Can you work these out from the model? Positions are in its coordinate system, mm. A direction names the side the tool comes from. Round coordinates to 2 decimals unless told otherwise and drop trailing zeros. Order: outer loops, then holes, each group sorted by start corner. A loop starts at its lowest first (then second) coordinate and runs counter-clockwise, first axis right, second up.
Q1. Will these pins go through, and if not, where does the flat tip stop? P1, Ø2, axis at x = -15, z = 0, coming from the -Y side; P2, Ø4, axis at x = 22, z = 0, coming from the -Y side; P3, Ø3, axis at x = -20.5, z = 0.5, coming from the -Y side; P4, Ø5, axis at x = -12, z = 24, coming from the -Y side.
Q2. We'd pull the mould along Z, two halves only. Please class faces 1 (the face through (-9, 18.5, -13)), 2 (the face through (-12, -17, 0)): pulls with the +Z half, pulls with the -Z half, needs draft (parallel to the pull), parting line crosses it, or undercut.
Q3. For faces 3 (the face through (21.57, 17.49, -0.65)), 4 (the face through (-12.436, 15.451, 15.94)), 5 (the face through (-7, -15.5, 7)), which set-ups out of +Z, -Z, +X, -X, +Y, -Y let a thin tool reach every point of the face, with its end or its side?
Q4. If I drill on line 1 (Z direction, x = 0, y = -16); line 2 (Z direction, x = 10, y = 18.1); line 3 (Y direction, x = -12.5, z = 8), over which ranges is the centre line in solid material (lowest first)?
Q5. If we section it at C-C (y = -4): Please give me the cut outline in (x, z).
Q6. If we section it at B-B (x = 0): Please give me the cut outline in (y, z).
Q7. If we section it at D-D (z = -22): Count the separate pieces of the cut face and the enclosed holes in it, plus the area to 3 significant figures.
Q8. If we section it at A-A (y = 4.5): Please give me the cut outline in (x, z), plus the area to 3 significant figures.
from build123d import *

# Parameters (mm, degrees)
SKETCH_W              = 76
SKETCH_H              = 37
PAD_DEPTH             = 30
SKETCH020_R           = 14
POCKET_DEPTH          = 8
SKETCH026_R           = 1.7
PAD001_DEPTH          = 2
POCKET001_DEPTH       = 4
POLARPATTERN_COUNT    = 6
SKETCH025_R           = 1.7
POCKET005_DEPTH       = 211.317184
POLARPATTERN001_COUNT = 6
SKETCH022_R           = 1.7
SKETCH022_R_2         = 7
SKETCH022_W           = 3.5
SKETCH022_H           = 5
POCKET002_DEPTH       = 5
SKETCH027_W           = 5
SKETCH027_H           = 30
POCKET006_DEPTH       = 4.001
SKETCH028_R           = 1.6
POCKET007_DEPTH       = 5
POCKET008_DEPTH       = 2
FILLET_R              = 7
FILLET001_R           = 7
FILLET002_R           = 5
FILLET003_R           = 5
FILLET004_R           = 3
FILLET005_R           = 3
FILLET006_R           = 3
FILLET007_R           = 3
FILLET008_R           = 2
FILLET009_R           = 2
CHAMFER_SIZE          = 1.7
CHAMFER001_SIZE       = 1.7
CHAMFER002_SIZE       = 1.7
CHAMFER003_SIZE       = 1.7


with BuildPart() as part:
    # Sketch → Pad (new body, symmetric)
    with BuildSketch(Plane.XY):
        Rectangle(SKETCH_W, SKETCH_H)
        Polygon((-34, -11.5), (-30, -15.5), (30, -15.5), (34, -11.5), (34, 12.5), (12.5, 14.5), (-12.5, 14.5), (-34, 12.5), align=None, mode=Mode.SUBTRACT)
    extrude(amount=PAD_DEPTH, both=True)

    # Sketch020 → Pocket (cut)
    with BuildSketch(Plane(origin=(0, 18.5, 0), x_dir=(-1, 0, 0), z_dir=(0, 1, 0))):
        Circle(SKETCH020_R)
    extrude(amount=-POCKET_DEPTH, mode=Mode.SUBTRACT)

    # Sketch026 → Pad001 (new body)
    with BuildSketch(Plane.XZ.offset(-14.5)):
        with Locations((20, 0)):
            Circle(SKETCH026_R)
    extrude(amount=PAD001_DEPTH)

    # Sketch021 → Pocket001 (cut)
    with BuildSketch(Plane.XZ.offset(-12.5)):
        Polygon((18.383419, 2.8), (16.766838, 0), (18.383419, -2.8), (21.616581, -2.8), (23.233162, 0), (21.616581, 2.8), align=None)
    pocket001 = extrude(amount=-POCKET001_DEPTH, mode=Mode.SUBTRACT)

    # PolarPattern: Pocket001 ×6 about axis
    polarpattern_axis = Axis((0, 12.5, 0), (0, -1, 0))
    for i in range(1, POLARPATTERN_COUNT):
        add(pocket001.rotate(polarpattern_axis, i * 360 / POLARPATTERN_COUNT), mode=Mode.SUBTRACT)

    # Sketch025 → Pocket005 (cut, through all)
    with BuildSketch(Plane.XZ.offset(-14.5)):
        with Locations((20, 0)):
            Circle(SKETCH025_R)
    pocket005 = extrude(amount=-POCKET005_DEPTH, mode=Mode.SUBTRACT)

    # PolarPattern001: Pocket005 ×6 about axis
    polarpattern001_axis = Axis((0, 14.5, 0), (0, -1, 0))
    for i in range(1, POLARPATTERN001_COUNT):
        add(pocket005.rotate(polarpattern001_axis, i * 360 / POLARPATTERN001_COUNT), mode=Mode.SUBTRACT)

    # Sketch022 → Pocket002 (cut)
    with BuildSketch(Plane.XZ.offset(18.5)):
        with Locations((0, 22)):
            Circle(SKETCH022_R)
        with Locations((0, -22)):
            Circle(SKETCH022_R)
        with Locations((-22, 0)):
            Circle(SKETCH022_R)
        with Locations((22, 0)):
            Circle(SKETCH022_R)
        Circle(SKETCH022_R_2)
        with Locations((-15, 0)):
            Circle(SKETCH022_R)
        with BuildLine():
            ThreePointArc((-23.660997, 14.014536), (-21.731705, 6.47943), (-14.196598, 8.408722))
            ThreePointArc((-8.408722, 14.196598), (-11.667262, 11.667262), (-14.196598, 8.408722))
            ThreePointArc((-8.408722, 14.196598), (-6.47943, 21.731705), (-14.014536, 23.660997))
            ThreePointArc((-14.014536, 23.660997), (-19.445436, 19.445436), (-23.660997, 14.014536))
        make_face()
        with BuildLine():
            ThreePointArc((8.408722, -14.196598), (11.667262, -11.667262), (14.196598, -8.408722))
            ThreePointArc((23.660997, -14.014536), (21.731705, -6.47943), (14.196598, -8.408722))
            ThreePointArc((14.014536, -23.660997), (19.445436, -19.445436), (23.660997, -14.014536))
            ThreePointArc((8.408722, -14.196598), (6.47943, -21.731705), (14.014536, -23.660997))
        make_face()
        with BuildLine():
            ThreePointArc((23.660997, 14.014536), (19.445436, 19.445436), (14.014536, 23.660997))
            ThreePointArc((14.014536, 23.660997), (6.47943, 21.731705), (8.408722, 14.196598))
            ThreePointArc((14.196598, 8.408722), (11.667262, 11.667262), (8.408722, 14.196598))
            ThreePointArc((14.196598, 8.408722), (21.731705, 6.47943), (23.660997, 14.014536))
        make_face()
        with BuildLine():
            ThreePointArc((-14.014536, -23.660997), (-6.47943, -21.731705), (-8.408722, -14.196598))
            ThreePointArc((-14.196598, -8.408722), (-11.667262, -11.667262), (-8.408722, -14.196598))
            ThreePointArc((-14.196598, -8.408722), (-21.731705, -6.47943), (-23.660997, -14.014536))
            ThreePointArc((-23.660997, -14.014536), (-19.445436, -19.445436), (-14.014536, -23.660997))
        make_face()
        with Locations((-10.25, 0)):
            Rectangle(SKETCH022_W, SKETCH022_H)
    extrude(amount=-POCKET002_DEPTH, mode=Mode.SUBTRACT)

    # Sketch027 → Pocket006 (cut, through all)
    with BuildSketch(Plane.XZ.offset(-14.5)):
        with Locations((0, 15)):
            Rectangle(SKETCH027_W, SKETCH027_H)
    extrude(amount=-POCKET006_DEPTH, mode=Mode.SUBTRACT)

    # Sketch028 → Pocket007 (cut)
    with BuildSketch(Plane(origin=(-38, 0, 0), x_dir=(0, -1, 0), z_dir=(-1, 0, 0))):
        with Locations((4, 17.5)):
            Circle(SKETCH028_R)
        with Locations((4, -17.5)):
            Circle(SKETCH028_R)
        with BuildLine():
            ThreePointArc((11, 5), (4, 12), (-3, 5))
            Line((-3, 5), (-3, -5))
            ThreePointArc((-3, -5), (4, -12), (11, -5))
            Line((11, 5), (11, -5))
        make_face()
    extrude(amount=-POCKET007_DEPTH, mode=Mode.SUBTRACT)

    # Sketch029 → Pocket008 (cut)
    with BuildSketch(Plane.YZ.offset(-34)):
        Polygon((-2.383419, 14.7), (-0.766838, 17.5), (-2.383419, 20.3), (-5.616581, 20.3), (-7.233162, 17.5), (-5.616581, 14.7), align=None)
        Polygon((-7.233162, -17.5), (-5.616581, -20.3), (-2.383419, -20.3), (-0.766838, -17.5), (-2.383419, -14.7), (-5.616581, -14.7), align=None)
    extrude(amount=-POCKET008_DEPTH, mode=Mode.SUBTRACT)

    # Fillet
    fillet_edges = [part.edges().sort_by_distance(p)[0] for p in [
        (-38, -18.5, 0),
    ]]
    fillet(fillet_edges, radius=FILLET_R)

    # Fillet001
    fillet001_edges = [part.edges().sort_by_distance(p)[0] for p in [
        (38, -18.5, 0),
    ]]
    fillet(fillet001_edges, radius=FILLET001_R)

    # Fillet002
    fillet002_edges = [part.edges().sort_by_distance(p)[0] for p in [
        (-34, 12.5, 0),
    ]]
    fillet(fillet002_edges, radius=FILLET002_R)

    # Fillet003
    fillet003_edges = [part.edges().sort_by_distance(p)[0] for p in [
        (34, 12.5, 0),
    ]]
    fillet(fillet003_edges, radius=FILLET003_R)

    # Fillet004
    fillet004_edges = [part.edges().sort_by_distance(p)[0] for p in [
        (-30, -15.5, 0),
    ]]
    fillet(fillet004_edges, radius=FILLET004_R)

    # Fillet005
    fillet005_edges = [part.edges().sort_by_distance(p)[0] for p in [
        (30, -15.5, 0),
    ]]
    fillet(fillet005_edges, radius=FILLET005_R)

    # Fillet006
    fillet006_edges = [part.edges().sort_by_distance(p)[0] for p in [
        (34, -11.5, 0),
    ]]
    fillet(fillet006_edges, radius=FILLET006_R)

    # Fillet007
    fillet007_edges = [part.edges().sort_by_distance(p)[0] for p in [
        (-34, -11.5, 0),
    ]]
    fillet(fillet007_edges, radius=FILLET007_R)

    # Fillet008
    fillet008_edges = [part.edges().sort_by_distance(p)[0] for p in [
        (-2.5, 16.5, 13.774977),
    ]]
    fillet(fillet008_edges, radius=FILLET008_R)

    # Fillet009
    fillet009_edges = [part.edges().sort_by_distance(p)[0] for p in [
        (2.5, 16.5, 13.774977),
    ]]
    fillet(fillet009_edges, radius=FILLET009_R)

    # Chamfer
    chamfer_edges = [part.edges().sort_by_distance(p)[0] for p in [
        (-1.7, -18.5, 22),
    ]]
    chamfer(chamfer_edges, length=CHAMFER_SIZE)

    # Chamfer001
    chamfer001_edges = [part.edges().sort_by_distance(p)[0] for p in [
        (20.3, -18.5, 0),
    ]]
    chamfer(chamfer001_edges, length=CHAMFER001_SIZE)

    # Chamfer002
    chamfer002_edges = [part.edges().sort_by_distance(p)[0] for p in [
        (-23.7, -18.5, 0),
    ]]
    chamfer(chamfer002_edges, length=CHAMFER002_SIZE)

    # Chamfer003
    chamfer003_edges = [part.edges().sort_by_distance(p)[0] for p in [
        (-1.7, -18.5, -22),
    ]]
    chamfer(chamfer003_edges, length=CHAMFER003_SIZE)


solid = part.part
Solution:
1. P1: stops at y = 14.17
1. P2: stops at y = -17.1
1. P3: stops at y = -18.18
1. P4: stops at y = -18.5
2. face 1: needs draft
2. face 2: undercut
3. face 3: +Y
3. face 4: -Y
3. face 5: +Z, -Z
4. line 1: z = -30 to -23.7, -20.3 to -7, 7 to 20.3, 23.7 to 30
4. line 2: z = -30 to -19.02, -15.62 to -9.8, 9.8 to 15.62, 19.02 to 30
4. line 3: y = -18.5 to -15.5, 14.5 to 18.5
5. outline: (-38, -30) - (-34, -30) - (-34, -20.3) - (-36, -20.3) - (-36, -19.1) - (-38, -19.1) - close; (-38, -15.9) - (-36, -15.9) - (-36, -14.7) - (-34, -14.7) - (-34, -12) - (-38, -12) - close; (-38, 12) - (-34, 12) - (-34, 14.7) - (-36, 14.7) - (-36, 15.9) - (-38, 15.9) - close; (-38, 19.1) - (-36, 19.1) - (-36, 20.3) - (-34, 20.3) - (-34, 30) - (-38, 30) - close; (34, -30) - (38, -30) - (38, 30) - (34, 30) - close
6. outline: (-18.5, -30) - (-15.5, -30) - (-15.5, -23.7) - (-16.8, -23.7) - (-18.5, -25.4) - close; (-18.5, -18.6) - (-16.8, -20.3) - (-15.5, -20.3) - (-15.5, -7) - (-18.5, -7) - close; (-18.5, 7) - (-15.5, 7) - (-15.5, 20.3) - (-16.8, 20.3) - (-18.5, 18.6) - close; (-18.5, 25.4) - (-16.8, 23.7) - (-15.5, 23.7) - (-15.5, 30) - (-18.5, 30) - close; (14.5, -30) - (18.5, -30) - (18.5, -14) - (14.5, -14) - close
7. separate pieces: 3
7. enclosed holes: 0
7. area: 747 mm2
8. outline: (-38, -30) - (-34, -30) - (-34, 30) - (-38, 30) - close; (34, -30) - (38, -30) - (38, 30) - (34, 30) - close
8. area: 480 mm2
